Here's how the part is built. I have some questions about the finished solid (model axes, mm). Face numbers are marked on the shaded views. A direction names the side the tool comes from. Round coordinates to 2 decimals unless told otherwise and drop trailing zeros. Order: outer loops, then holes, each group sorted by start corner. A loop starts at its lowest first (then second) coordinate and runs counter-clockwise, first axis right, second up.
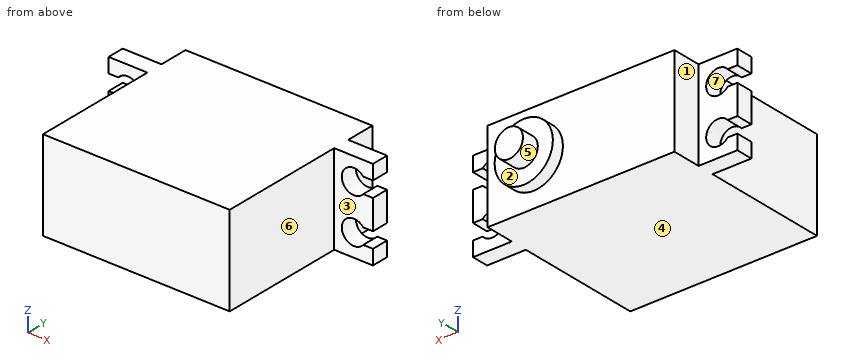
```python
from build123d import *

# Parameters (mm, degrees)
BOSS_EXTRU_1_DEPTH      = 18.5
ENL_V_MAT_EXTRU_1_DEPTH = 58.017897583
ESQUISSE4_W             = 38.5
ESQUISSE4_H             = 18.5
BOSS_EXTRU_2_DEPTH      = 6
ESQUISSE6_R             = 6
BOSS_EXTRU_3_DEPTH      = 2.5
ESQUISSE7_R             = 2.9
BOSS_EXTRU_4_DEPTH      = 3.7


with BuildPart() as part:
    # Esquisse2 → Boss.-Extru.1 (new body)
    with BuildSketch(Plane.XY):
        Polygon((-9.349799062, -0.125566913), (-9.349799062, 3.374433087), (45.150200938, 3.374433087), (45.150200938, -0.125566913), (37.150200938, -0.125566913), (37.150200938, -26.125566913), (-1.349799062, -26.125566913), (-1.349799062, -0.125566913), align=None)
    extrude(amount=BOSS_EXTRU_1_DEPTH)

    # Esquisse3 → Enlèv. mat.-Extru.1 (cut, through all)
    with BuildSketch(Plane(origin=(0, 3.374433087, 0), x_dir=(1, 0, 0), z_dir=(0, 1, 0))):
        with BuildLine():
            Line((-9.349799062, -15.468288585), (-7.349799062, -15.468288585))
            ThreePointArc((-7.349799062, -15.468288585), (-2.923291475, -13.875), (-7.349799062, -12.281711415))
            Line((-7.349799062, -12.281711415), (-9.349799062, -12.281711415))
            Line((-9.349799062, -12.281711415), (-9.349799062, -15.468288585))
        make_face()
        with BuildLine():
            Line((45.150200938, -12.281711415), (43.150200938, -12.281711415))
            ThreePointArc((43.150200938, -12.281711415), (38.723693351, -13.875), (43.150200938, -15.468288585))
            Line((43.150200938, -15.468288585), (45.150200938, -15.468288585))
            Line((45.150200938, -15.468288585), (45.150200938, -12.281711415))
        make_face()
        with BuildLine():
            Line((-9.349799062, -6.218288585), (-7.349799062, -6.218288585))
            ThreePointArc((-7.349799062, -6.218288585), (-2.923291475, -4.625), (-7.349799062, -3.031711415))
            Line((-7.349799062, -3.031711415), (-9.349799062, -3.031711415))
            Line((-9.349799062, -3.031711415), (-9.349799062, -6.218288585))
        make_face()
        with BuildLine():
            Line((45.150200938, -3.031711415), (43.150200938, -3.031711415))
            ThreePointArc((43.150200938, -3.031711415), (38.723693351, -4.625), (43.150200938, -6.218288585))
            Line((43.150200938, -6.218288585), (45.150200938, -6.218288585))
            Line((45.150200938, -6.218288585), (45.150200938, -3.031711415))
        make_face()
    extrude(amount=-ENL_V_MAT_EXTRU_1_DEPTH, mode=Mode.SUBTRACT)

    # Esquisse4 → Boss.-Extru.2 (add)
    with BuildSketch(Plane(origin=(0, 3.374433087, 0), x_dir=(1, 0, 0), z_dir=(0, 1, 0))):
        with Locations((17.900200938, -9.25)):
            Rectangle(ESQUISSE4_W, ESQUISSE4_H)
    extrude(amount=BOSS_EXTRU_2_DEPTH)

    # Esquisse6 → Boss.-Extru.3 (add)
    with BuildSketch(Plane(origin=(0, 9.374433087, 0), x_dir=(1, 0, 0), z_dir=(0, 1, 0))):
        with Locations(Location((27.650200938, -9.25, 0), (0, 0, 270))):
            Circle(ESQUISSE6_R)
    extrude(amount=BOSS_EXTRU_3_DEPTH)

    # Esquisse7 → Boss.-Extru.4 (add)
    with BuildSketch(Plane(origin=(0, 11.874433087, 0), x_dir=(1, 0, 0), z_dir=(0, 1, 0))):
        with Locations(Location((27.650200938, -9.25, 0), (0, 0, 270))):
            Circle(ESQUISSE7_R)
    extrude(amount=BOSS_EXTRU_4_DEPTH)


solid = part.part
```
1) I need wall thicknesses on line 1 (Y direction, x = 34.5, z = 4.5); line 2 (Y direction, x = 38, z = 3.5); line 3 (X direction, y = -23.5, z = 2). Which ranges of each line are inside material? Lowest first, please.
2) If we section it at B-B (x = 14.5): Write out the boundary of the cut face in (y, z).
3) If we section it at C-C (y = -13): Write out the boundary of the cut face in (x, z).
4) I'm going to push flat-ended pins straight in: pin 1 (1.8 mm diameter, centred on y = 7, z = 9.5, fed in from -X); pin 2 (10 mm diameter, centred on x = 1, z = 5, fed in from +Y); pin 3 (1.8 mm diameter, centred on y = 7, z = 8.5, fed in from +X). Where does each tip first touch, or does it pass through?
5) If we section it at A-A (z = 9.25): Write out the boundary of the cut face in (x, y), plus the area to 3 significant figures.
6) If we section it at D-D (z = 5.5): Write out the boundary of the cut face in (x, y).
7) We'd pull the mould along Z, two halves only. Please class the marked faces 4, 5, 6 and 7: +Z half, -Z half, draft (parallel to the pull), parting line (faces both ways), or undercut.
8) For the marked faces 1, 2 and 3, which set-ups out of +Z, -Z, +X, -X, +Y, -Y let a thin tool reach every point of the face, with its end or its side?
Solutions:
1. line 1: y = -26.13 to 9.37
1. line 2: y = -0.13 to 3.37
1. line 3: x = -1.35 to 37.15
2. outline: (-26.13, 0) - (9.37, 0) - (9.37, 18.5) - (-26.13, 18.5) - close
3. outline: (-1.35, 0) - (37.15, 0) - (37.15, 18.5) - (-1.35, 18.5) - close
4. pin 1: stops at x = -1.35
4. pin 2: stops at y = 9.37
4. pin 3: stops at x = 37.15
5. outline: (-9.35, -0.13) - (-1.35, -0.13) - (-1.35, -26.13) - (37.15, -26.13) - (37.15, -0.13) - (45.15, -0.13) - (45.15, 3.37) - (37.15, 3.37) - (37.15, 9.37) - (33.65, 9.37) - (33.65, 11.87) - (30.55, 11.87) - (30.55, 15.57) - (24.75, 15.57) - (24.75, 11.87) - (21.65, 11.87) - (21.65, 9.37) - (-1.35, 9.37) - (-1.35, 3.37) - (-9.35, 3.37) - close
5. area: 1,470 mm2
6. outline: (-3.08, -0.13) - (-1.35, -0.13) - (-1.35, -26.13) - (37.15, -26.13) - (37.15, -0.13) - (38.88, -0.13) - (38.88, 3.37) - (37.15, 3.37) - (37.15, 9.37) - (32.33, 9.37) - (32.33, 11.87) - (22.97, 11.87) - (22.97, 9.37) - (-1.35, 9.37) - (-1.35, 3.37) - (-3.08, 3.37) - close
7. face 4: -Z half
7. face 5: parting line
7. face 6: draft
7. face 7: undercut
8. face 1: +Z, -Z, -X, +Y
8. face 2: +Y
8. face 3: +Z, -Z, +X, -Y
